Autodesk Inventor part; units mm, degrees
ref_plane "YZ Plane" through (0, 0, 0) normal (1, 0, 0) x (0, 1, 0)
ref_plane "XZ Plane" through (0, 0, 0) normal (0, 1, 0) x (-1, 0, 0)
ref_plane "XY Plane" through (0, 0, 0) normal (0, 0, 1) x (1, 0, 0)
sketch "Sketch1" plane through (0, 0, 0) normal (1, 0, 0) x (0, 1, 0)
  line L0 (7.5884, 18.4529) -> (-11.4616, 18.4529)
  line L1 (-11.4616, 18.4529) -> (-11.4616, -33.6171)
  line L2 (-11.4616, -33.6171) -> (7.5884, -33.6171)
  line L3 (7.5884, -33.6171) -> (7.5884, 18.4529)
  point P0 (0, 0)
  dimension "d0" = 52.07
  dimension "d1" = 19.05
extrude "Extrusion1" add sketch "Sketch1" along normal blind 6.35
sketch "Sketch3" plane through (0, 7.5884, 18.4529) normal (0, 1, 0) x (1, 0, 0)
  line L0 (0, 26.67) -> (0.635, 26.67)
  line L1 (0.635, 26.67) -> (0.635, 52.07)
  line L2 (0.635, 52.07) -> (0, 52.07)
  line L3 (0, 52.07) -> (0, 26.67)
  line L4 (5.715, 52.07) -> (6.35, 52.07)
  line L5 (6.35, 52.07) -> (6.35, 26.67)
  line L6 (6.35, 26.67) -> (5.715, 26.67)
  line L7 (5.715, 26.67) -> (5.715, 52.07)
  line L8 (6.35, 52.07) -> (6.35, 0)
  line L9 (0, 52.07) -> (0, 0)
  line L10 (0, 52.07) -> (6.35, 52.07)
  point P0 (0, 18.4529)
  dimension "d19" = 25.4
  dimension "d20" = 25.4
  dimension "d21" = 0
  dimension "d22" = 0
  dimension "d23" = 0.635
  dimension "d24" = 0.635
  dimension "d25" = 0
extrude "Extrusion2" cut sketch "Sketch3" against normal blind 50.8
sketch "Sketch4" plane through (0, 7.5884, 18.4529) normal (0, 1, 0) x (1, 0, 0)
  line L0 (0.635, 34.7601) -> (-3.8704, 34.7601)
  line L1 (-3.8704, 34.7601) -> (-3.8704, -3.0853)
  line L2 (-3.8704, -3.0853) -> (0.635, -3.0853)
  line L3 (0.635, -3.0853) -> (0.635, 34.7601)
  line L4 (0.635, 52.07) -> (0.635, 26.67)
  point P0 (0, 18.4529)
  dimension "d28" = 0
extrude "Extrusion3" cut sketch "Sketch4" against normal blind 25.4
sketch "Sketch5" plane through (0.635, 7.5884, -33.6171) normal (-1, 0, 0) x (0, 0, 1)
  line L0 (52.07, 0) -> (52.07, -19.05)
  line L1 (0, 0) -> (52.07, 0)
  line L2 (0, -19.05) -> (0, 0)
  point P0 (33.6171, -7.5884)
  point P1 (45.72, -6.35)
  point P2 (33.02, -12.7)
  point P3 (12.7, -5.08)
  point P4 (12.7, -13.97)
  dimension "d31" = 6.35
  dimension "d32" = 6.35
  dimension "d33" = 12.7
  dimension "d34" = 19.05
  dimension "d35" = 5.08
  dimension "d36" = 12.7
  dimension "d37" = 12.7
  dimension "d38" = 13.97
hole "Hole2" at (0.635, 1.2384, 12.1029) at (0.635, -5.1116, -0.5971) at (0.635, 2.5084, -20.9171) at (0.635, -6.3816, -20.9171) direction (1, 0, 0) diameter 4.4958 end through all countersink diameter 8.4328 countersink angle 82
properties part number "SidePlate"
Could you check a few things on this model? Use its own coordinates, in mm. Round coordinates to 2 decimals unless told otherwise and drop trailing zeros. Order: outer loops, then holes, each group sorted by start corner. A loop starts at its lowest first (then second) coordinate and runs counter-clockwise, first axis right, second up.
Q1. Please list where these lines run through material, in increasing order: probe 1 along Z at (x, y) = (3.2, -4.5); probe 2 along Z at (x, y) = (3.65, 2); probe 3 along Y at (x, z) = (2.45, -22.5).
Geometry says:
probe 1: z = -33.62 to -22.15, -19.69 to -2.76, 1.57 to 18.45
probe 2: z = -33.62 to -23.11, -18.73 to 9.99, 14.22 to 18.45
probe 3: y = -11.46 to -8.49, -4.27 to 0.4, 4.62 to 7.59
Q2. Imagine slicing it at A-A, the plane x = 4.7. List the corners of the cut face in (y, z) for me.
Geometry says:
outline: (-11.46, -33.62) - (7.59, -33.62) - (7.59, 18.45) - (-11.46, 18.45) - close; hole circle Ø4.5 at (-6.38, -20.92); hole circle Ø4.5 at (-5.11, -0.6); hole circle Ø4.5 at (1.24, 12.1); hole circle Ø4.5 at (2.51, -20.92)
Q3. I'm going to push flat-ended pins straight in: P1, Ø6, axis at y = -5.11, z = -0.6, coming from the -X side; P2, Ø0.5, axis at x = 6, y = 0, coming from the -Z side. Where does each tip first touch, or does it pass through?
Geometry says:
P1: stops at x = 2.03
P2: stops at z = -8.22
Q4. Thinking about a two-plate mould opening in Z: for faces 1 (the face through (5.715, -2, -21)), 2 (the face through (3, -2, -33.617)), 3 (the face through (2.758, -4.031, -21.226)), 4 (the face through (2.76, 1.95, 14.36)), which applies, released by +Z, released by -Z, zero draft, split by the parting line, or undercut?
Geometry says:
face 1: zero draft
face 2: released by -Z
face 3: undercut
face 4: undercut
Q5. Imagine slicing it at B-B, the plane z = -15. List the corners of the cut face in (x, y) for me (3 decimals), then the cut area to 3 significant figures.
Geometry says:
outline: (0.635, -11.462) - (5.715, -11.462) - (5.715, 7.588) - (0.635, 7.588) - close
area: 96.8 mm2
Q6. Imagine slicing it at C-C, the plane y = 2. State how many separate pieces and enclosed holes the cut face has, then the cut area to 3 significant figures.
Geometry says:
separate pieces: 3
enclosed holes: 0
area: 226 mm2
Q7. Imagine slicing it at D-D, the plane x = 1.9. List the corners of the cut face in (y, z) for me.
Geometry says:
outline: (-11.46, -33.62) - (7.59, -33.62) - (7.59, 18.45) - (-11.46, 18.45) - close; hole circle Ø6.23 at (-6.38, -20.92); hole circle Ø6.23 at (-5.11, -0.6); hole circle Ø6.23 at (1.24, 12.1); hole circle Ø6.23 at (2.51, -20.92)
